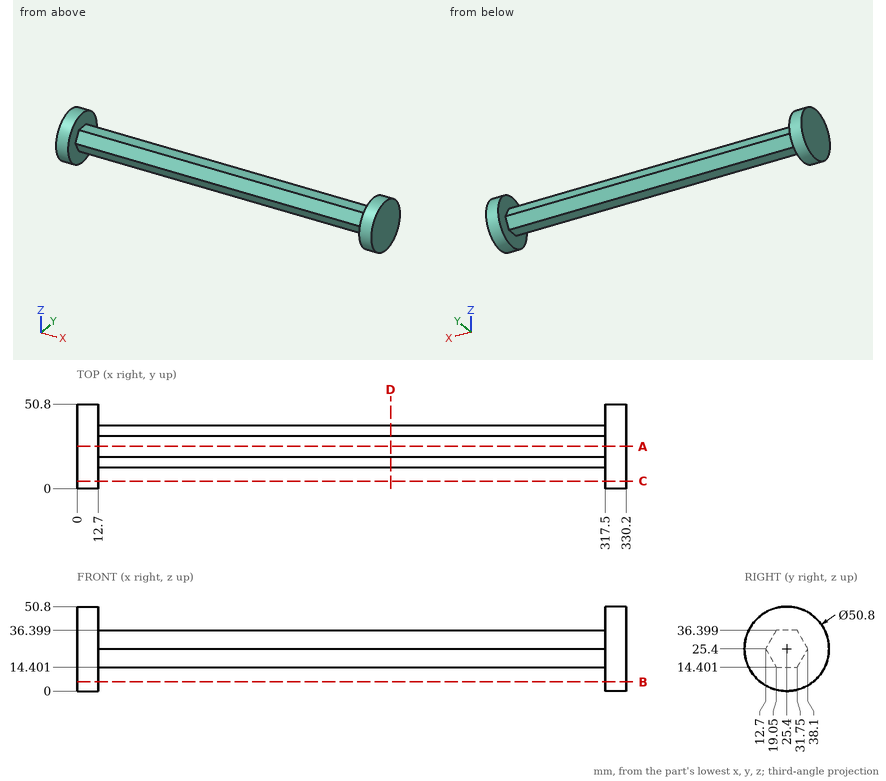
Design review of the part shown in the three views and the two pictorial views. Dimensions are in mm from the part's minimum x, y and z. Round coordinates to 2 decimals unless told otherwise and drop trailing zeros. Loops run counter-clockwise (first coordinate to the right, second up) from the corner with the lowest first, then second, coordinate; pieces in that order, holes last.
(1) We need section A-A (y = 25.4). Give the boundary of the cut face in (x, z).
Returned:
outline: (0, 0) - (12.7, 0) - (12.7, 14.4) - (317.5, 14.4) - (317.5, 0) - (330.2, 0) - (330.2, 50.8) - (317.5, 50.8) - (317.5, 36.4) - (12.7, 36.4) - (12.7, 50.8) - (0, 50.8) - close
(2) We need section C-C (y = 4.5). Give the boundary of the cut face in (x, z) (1 decimal).
Returned:
outline: (0, 11) - (12.7, 11) - (12.7, 39.8) - (0, 39.8) - close; (317.5, 11) - (330.2, 11) - (330.2, 39.8) - (317.5, 39.8) - close
(3) We need section B-B (z = 5.5). Give the boundary of the cut face in (x, y) (1 decimal).
Returned:
outline: (0, 9.6) - (12.7, 9.6) - (12.7, 41.2) - (0, 41.2) - close; (317.5, 9.6) - (330.2, 9.6) - (330.2, 41.2) - (317.5, 41.2) - close
(4) Clearance check with flat-ended pins moving along their axes: P1, Ø6.5, axis at x = 181.5, y = 23, coming from the -Z side; P2, Ø4, axis at x = 197.5, y = 25, coming from the +Z side; P3, Ø1, axis at x = 294, z = 27.5, coming from the -Y side (1 decimal). State where each tip first meets the part, or that it passes through.
Returned:
P1: stops at z = 14.4
P2: stops at z = 36.4
P3: stops at y = 13.6
(5) We need section D-D (x = 188.5). Give the boundary of the cut face in (y, z).
Returned:
outline: (12.7, 25.4) - (19.05, 14.4) - (31.75, 14.4) - (38.1, 25.4) - (31.75, 36.4) - (19.05, 36.4) - close
(6) Wall thickness on line 1 along X through (y, z) = (41, 9); line 2 along Z through (x, y) = (170, 21.5): over which ranges is each line inside the solid? List them lowest first.
Returned:
line 1: x = 0 to 12.7, 317.5 to 330.2
line 2: z = 14.4 to 36.4
